For this review, use the dimensioned drawing (mm, ordinates from the lowest corner) and the shaded views. Coordinates: 2 decimals unless noted, no trailing zeros. Order: outer loops, then holes, each group sorted by start corner. A loop starts at its lowest first (then second) coordinate and runs counter-clockwise, first axis right, second up. Notation, with made-up numbers: (-35.75, -35) -> (-24.75, -35) arc R22 ccw to (-24.75, -2) -> close; hole circle Ø6 at (59, 69.5). An arc over 180 degrees is marked (long way). Return JSON: item names as keys, results as strings. Group by question number.
Item 1: Take a section at B-B (z = 15). Write out the cut boundary in (x, y), then the cut area to 3 significant figures.
Item 2: For line 1 along Y through (x, z) = (5.4, 12.5); line 2 along Y through (x, z) = (1.95, 22.25); line 3 along Z through (x, y) = (2.9, 6.5), list the stretches that pass through material, from the lowest coordinate up.
Item 3: Insertion check: pin 1 (4 mm diameter, centred on y = 5.5, z = 15, fed in from +X); pin 2 (1.5 mm diameter, centred on x = 2.5, y = 6.5, fed in from -Z); pin 3 (1.5 mm diameter, centred on y = 6, z = 18.5, fed in from +X). Each pin has a flat end and moves straight along its axis. Give the tip position at first contact, or say it passes through.
Item 4: Take a section at A-A (x = 3). Write out the cut boundary in (y, z), then the cut area to 3 significant figures.
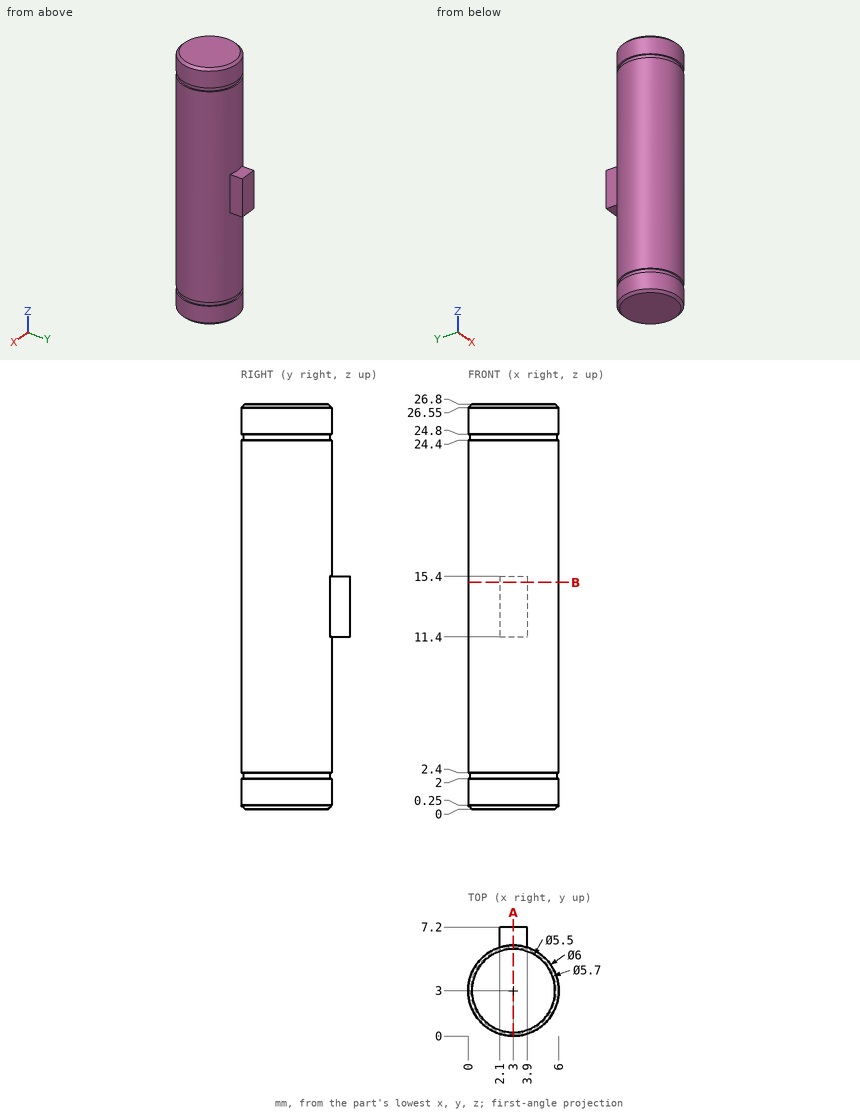
Findings below:
{
 "1": {"outline": "(2.1, 5.86) arc R3 ccw (long way) to (3.9, 5.86) -> (3.9, 7.2) -> (2.1, 7.2) -> close", "area": "30.5 mm2"},
 "2": {"line 1": "y = 1.2 to 4.8", "line 2": "y = 0.19 to 5.81", "line 3": "z = 11.4 to 15.4"},
 "3": {"pin 1": "stops at x = 5.96", "pin 2": "stops at z = 0.04", "pin 3": "stops at x = 4.98"},
 "4": {"outline": "(0, 0.25) -> (0.25, 0) -> (5.75, 0) -> (6, 0.25) -> (6, 2) -> (5.85, 2) -> (5.85, 2.4) -> (6, 2.4) -> (6, 11.4) -> (7.2, 11.4) -> (7.2, 15.4) -> (6, 15.4) -> (6, 24.4) -> (5.85, 24.4) -> (5.85, 24.8) -> (6, 24.8) -> (6, 26.55) -> (5.75, 26.8) -> (0.25, 26.8) -> (0, 26.55) -> (0, 24.8) -> (0.15, 24.8) -> (0.15, 24.4) -> (0, 24.4) -> (0, 2.4) -> (0.15, 2.4) -> (0.15, 2) -> (0, 2) -> close", "area": "165 mm2"}
}
